Work out the finished part from the listing and answer in its coordinate system (mm). Give positions to 0.01 mm unless a question says otherwise; leave off trailing zeros. Loops run counter-clockwise (first coordinate to the right, second up) from the corner with the lowest first, then second, coordinate; pieces in that order, holes last. Notation, with made-up numbers: (37, 3) -> (82, 3) arc R12 ccw to (82, 13) -> close; hole circle Ø2 at (27.5, 41). An arc over 180 degrees is marked (long way). Answer as CSV lines item,"result". Start each with the question number.
1. Find section C-C, the plane y = 10. Give the vertices of the cut face in (x, z), and give its area (4 significant figures).
2. Find section A-A, the plane x = 70. Give the vertices of the cut face in (y, z), and give its area (3 significant figures).
3. Find section B-B, the plane y = 145. Give the vertices of the cut face in (x, z), and give its area (3 significant figures).
4. Find section D-D, the plane x = 50. Give the vertices of the cut face in (y, z).
5. Find the intervals of material crossed by line 1 along X through (y, z) = (145, 3.7); line 2 along Y through (x, z) = (170, 1.4); line 3 along X through (y, z) = (10.5, 2.1), in increasing order.
from build123d import *

# Parameters (mm, degrees)
SKETCH1_W           = 180
SKETCH1_H           = 155
BOSS_EXTRUDE1_DEPTH = 5
SKETCH2_R           = 25
CUT_EXTRUDE1_DEPTH  = 6
SKETCH3_R           = 3.25
SKETCH3_R_2         = 2.65
CUT_EXTRUDE2_DEPTH  = 6


with BuildPart() as part:
    # Sketch1 → Boss-Extrude1 (new body)
    with BuildSketch(Plane.XY):
        with Locations((90, 77.5)):
            Rectangle(SKETCH1_W, SKETCH1_H)
    extrude(amount=BOSS_EXTRUDE1_DEPTH)

    # Sketch2 → Cut-Extrude1 (cut, through all)
    with BuildSketch(Plane.XY.offset(5)):
        with Locations((90, 67)):
            Circle(SKETCH2_R)
    extrude(amount=-CUT_EXTRUDE1_DEPTH, mode=Mode.SUBTRACT)

    # Sketch3 → Cut-Extrude2 (cut, through all)
    with BuildSketch(Plane.XY.offset(5)):
        with Locations((110, 101.641016151)):
            Circle(SKETCH3_R)
        with Locations((130, 67)):
            Circle(SKETCH3_R)
        with Locations((110, 32.358983849)):
            Circle(SKETCH3_R)
        with Locations((70, 32.358983849)):
            Circle(SKETCH3_R)
        with Locations((50, 67)):
            Circle(SKETCH3_R)
        with Locations((70, 101.641016151)):
            Circle(SKETCH3_R)
        with Locations((10, 145)):
            Circle(SKETCH3_R_2)
        with Locations((10, 77.5)):
            Circle(SKETCH3_R_2)
        with Locations((10, 10)):
            Circle(SKETCH3_R_2)
        with Locations((170, 10)):
            Circle(SKETCH3_R_2)
        with Locations((170, 77.5)):
            Circle(SKETCH3_R_2)
        with Locations((170, 145)):
            Circle(SKETCH3_R_2)
        with Locations((90, 10)):
            Circle(SKETCH3_R_2)
    extrude(amount=-CUT_EXTRUDE2_DEPTH, mode=Mode.SUBTRACT)


solid = part.part
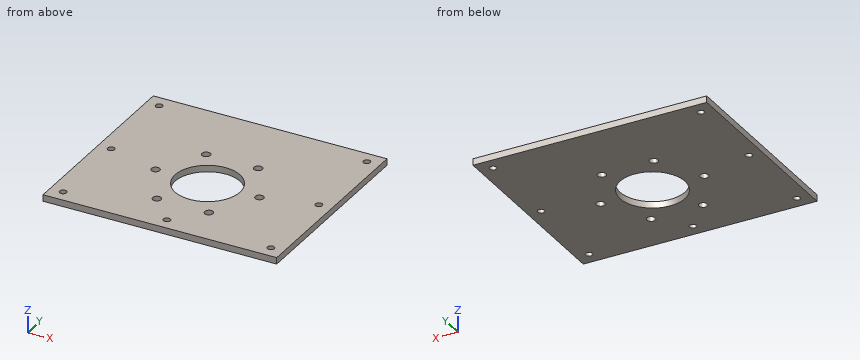
Resolved:
1,outline,"(0, 0) -> (7.35, 0) -> (7.35, 5) -> (0, 5) -> close; (12.65, 0) -> (87.35, 0) -> (87.35, 5) -> (12.65, 5) -> close; (92.65, 0) -> (167.35, 0) -> (167.35, 5) -> (92.65, 5) -> close; (172.65, 0) -> (180, 0) -> (180, 5) -> (172.65, 5) -> close"
1,area,"820.5 mm^2"
2,outline,"(0, 0) -> (29.11, 0) -> (29.11, 5) -> (0, 5) -> close; (35.61, 0) -> (52, 0) -> (52, 5) -> (35.61, 5) -> close; (82, 0) -> (98.39, 0) -> (98.39, 5) -> (82, 5) -> close; (104.89, 0) -> (155, 0) -> (155, 5) -> (104.89, 5) -> close"
2,area,"560 mm^2"
3,outline,"(0, 0) -> (7.35, 0) -> (7.35, 5) -> (0, 5) -> close; (12.65, 0) -> (167.35, 0) -> (167.35, 5) -> (12.65, 5) -> close; (172.65, 0) -> (180, 0) -> (180, 5) -> (172.65, 5) -> close"
3,area,"847 mm^2"
4,outline,"(0, 0) -> (63.75, 0) -> (63.75, 5) -> (0, 5) -> close; (70.25, 0) -> (155, 0) -> (155, 5) -> (70.25, 5) -> close"
5,line 1,"x = 0 to 7.35, 12.65 to 167.35, 172.65 to 180"
5,line 2,"y = 0 to 7.35, 12.65 to 74.85, 80.15 to 142.35, 147.65 to 155"
5,line 3,"x = 0 to 7.4, 12.6 to 87.4, 92.6 to 167.4, 172.6 to 180"
